Could you check a few things on this model? Use its own coordinates, in mm. A direction names the side the tool comes from. Give positions to 0.01 mm unless a question says otherwise; leave off trailing zeros. Loops run counter-clockwise (first coordinate to the right, second up) from the corner with the lowest first, then second, coordinate; pieces in that order, holes last. Notation, with made-up numbers: M -30.75,51 L 21.25,51 A11 cw 21.25,71 Z; hole C 89.25,24.25 d9. An arc over 180 degrees is marked long. Use a Markdown table: item, result. Add a question column.
1) Suppose I cut it at A-A on x = -154.5. List the corners of the cut face in (y, z) for me.
2) If I drill on line 1 along Z through (x, y) = (13, -159.5); line 2 along X through (y, z) = (7, 715); line 3 along X through (y, z) = (5.5, 314), over which ranges is the centre line in solid material (lowest first)? Write a range as [from, to].
3) Which directions (+Z, -Z, +X, -X, +Y, -Y) give clear straight access to the entire face, cutting with the end or side of a thin tool? Please do faces 1 (the cylindrical face through (-105.862, 81.172, 478.49)), 2 (the cylindrical face through (213.594, 212.972, 10.14)).
4) Will these pins go through, and if not, where does the flat tip stop? pin 1 Ø4 at (x, z) = (-67.5, 639.5) entering from -Y; pin 2 Ø1 at (x, z) = (73, 275) entering from -Y; pin 3 Ø8 at (y, z) = (-17, 836.5) entering from +X.
5) Suppose I cut it at C-C on y = 0. List the corners of the cut face in (x, z) for me, and give its area (3 significant figures).
Autodesk Fusion 360 part; units mm, degrees
sketch "Sketch1" plane through (0, 0, 0) normal (0, 0, 1) x (1, 0, 0)
  line L0 (225, 225) -> (-225, 225)
  line L1 (-225, 225) -> (-225, -225)
  line L2 (-225, -225) -> (225, -225)
  line L3 (225, -225) -> (225, 225)
  line L4 (225, 225) -> (-225, -225) construction
  line L5 (-225, 225) -> (225, -225) construction
  circle A0 centre (0, 0) radius 133.4
  dimension "d1" = 450
  dimension "d2" = 450
  dimension "d3" = 266.8
extrude "Extrude1" add sketch "Sketch1" along normal blind 20
extrude "Extrude2" add sketch "Sketch1" along normal blind 970 contours A0
sketch "Sketch2" plane through (0, 0, 970) normal (0, 0, 1) x (-1, 0, 0)
  circle A0 centre (0, 0) radius 133.4
  line L0 (225, 225) -> (-225, 225)
  line L1 (-225, 225) -> (-225, -225)
  line L2 (-225, -225) -> (225, -225)
  line L3 (225, -225) -> (225, 225)
  line L4 (225, 225) -> (-225, -225) construction
  line L5 (-225, 225) -> (225, -225) construction
  dimension "d8" = 450
  dimension "d9" = 450
extrude "Extrude3" add sketch "Sketch2" against normal blind 20
fillet "Fillet1" radius 40 8 edges at (225, 225, 960) (225, -225, 960) (-225, -225, 960) (-225, 225, 960) (-225, 225, 10) (-225, -225, 10) (225, 225, 10) (225, -225, 10)
Answer block:
| question | item | result |
|---|---|---|
| 1 | outline | M -225,0 L 225,0 L 225,20 L -225,20 Z; M -225,950 L 225,950 L 225,970 L -225,970 Z |
| 2 | line 1 | z = [0, 20], [950, 970] |
| 2 | line 2 | x = [-133.22, 133.22] |
| 2 | line 3 | x = [-133.29, 133.29] |
| 3 | face 1 | none |
| 3 | face 2 | +Z, -Z, +X, +Y |
| 4 | pin 1 | stops at y = -116.21 |
| 4 | pin 2 | stops at y = -111.98 |
| 4 | pin 3 | stops at x = 132.77 |
| 5 | outline | M -225,0 L 225,0 L 225,20 L 133.4,20 L 133.4,950 L 225,950 L 225,970 L -225,970 L -225,950 L -133.4,950 L -133.4,20 L -225,20 Z |
| 5 | area | 266,000 mm^2 |
